Part model, mm, in its own coordinate system. A direction names the side the tool comes from. Coordinates: 2 decimals unless noted, no trailing zeros. Order: outer loops, then holes, each group sorted by start corner. A loop starts at its lowest first (then second) coordinate and runs counter-clockwise, first axis right, second up.
from build123d import *

# Parameters (mm, degrees)
SKETCH1_R               = 76.2
SKETCH1_R_2             = 69.85
BOSS_EXTRUDE1_DEPTH     = 25.4
CUT_EXTRUDE1_REACH      = 112.716
CUT_EXTRUDE1_END_RADIUS = 76.2
SKETCH4_W               = 36.83
SKETCH4_H               = 7.62
FILLET1_R               = 2.54


with BuildPart() as part:
    # Sketch1 → Boss-Extrude1 (new, symmetric)
    with BuildSketch(Plane(origin=(0, 0, 0), x_dir=(0, 0, -1), z_dir=(1, 0, 0))):
        Circle(SKETCH1_R)
        Circle(SKETCH1_R_2, mode=Mode.SUBTRACT)
    extrude(amount=BOSS_EXTRUDE1_DEPTH, both=True)

    # Cut-Extrude1: up to this cylinder (the profile starts inside it)
    cut_extrude1_end = Plane(origin=(0, 0, 0), z_dir=(-1, 0, 0)) * Cylinder(CUT_EXTRUDE1_END_RADIUS, 378.832, mode=Mode.PRIVATE)
    # Sketch4 → Cut-Extrude1 (cut, up to the surface)
    with BuildSketch(Plane.XY, mode=Mode.PRIVATE) as cut_extrude1_sk1:
        with Locations((0, 62.865)):
            Rectangle(SKETCH4_W, SKETCH4_H)
    cut_extrude1_tool1 = extrude(cut_extrude1_sk1.sketch, amount=-CUT_EXTRUDE1_REACH, mode=Mode.PRIVATE) & cut_extrude1_end
    add(cut_extrude1_tool1.solids().sort_by_distance((0, 62.865, 0))[0], mode=Mode.SUBTRACT)

    # Fillet1
    fillet1_edges = [part.edges().sort_by_distance(p)[0] for p in [
        (-18.415, 59.055, -42.729327968),
        (-18.415, 66.675, -28.855016844),
        (18.415, 66.675, -28.855016844),
        (18.415, 59.055, -42.729327968),
    ]]
    fillet(fillet1_edges, radius=FILLET1_R)


solid = part.part
Q1. Which spindle directions (+Z, -Z, +X, -X, +Y, -Y) get a long thin tool onto all of the face, cutting with end or side? Do faces 1 (the face through (0, 59.055, -43)), 2 (the face through (-0.356, -42.503, 55.431)). Say none if no direction does.
Results list:
face 1: -Z, +Y
face 2: +X, -X
Q2. Cut at A-A on z = 0. Write the cut outline in (x, y), and give its area (3 significant figures).
Results list:
outline: (-25.4, -76.2) - (25.4, -76.2) - (25.4, -69.85) - (-25.4, -69.85) - close; (-25.4, 69.85) - (25.4, 69.85) - (25.4, 76.2) - (-25.4, 76.2) - close
area: 645 mm2
Q3. Mould opens along Y. For faces 3 (the face through (0.356, -74.388, 16.519)), 4 (the face through (0, 66.675, -29)), 5 (the face through (25.4, -62, -34)) say: pulls with the +Y half, pulls with the -Y half, needs draft (parallel to the pull), parting line crosses it, or undercut.
Results list:
face 3: parting line crosses it
face 4: undercut
face 5: needs draft
Q4. Wall check: line 1 along Y through (x, z) = (12, 0); line 2 along Z through (x, y) = (10.5, 1.5); line 3 along Z through (x, y) = (-6.5, -46). Give the ranges that are in metal, low to high.
Results list:
line 1: y = -76.2 to -69.85, 69.85 to 76.2
line 2: z = -76.19 to -69.83, 69.83 to 76.19
line 3: z = -60.75 to -52.56, 52.56 to 60.75
Q5. Pin check, flat tips, straight feed: pin 1 Ø5 at (x, z) = (5.5, -27.5) entering from -Y; pin 2 Ø10 at (x, y) = (-11.5, 25.5) entering from +Z; pin 3 Ø4 at (x, y) = (2, 4) entering from -Z. Stop position of each tip, or through.
Results list:
pin 1: stops at y = -71.98
pin 2: stops at z = 73.39
pin 3: stops at z = -76.17
Q6. Cut at C-C on x = -11. Write the cut outline in (y, z) (3 decimals), and give its area (3 significant figures).
Results list:
outline: (59.055, -48.155) - (59.055, -37.303) arc R69.85 cw (long way) to (66.675, -20.82) - (66.675, -36.89) arc R76.2 ccw (long way) to start
area: 2,820 mm2
